Study the drawing (mm; zero at the part's minimum x, y, z) and answer. Round coordinates to 2 decimals unless told otherwise and drop trailing zeros. Write each loop counter-clockwise with the first axis right and the second up, starting at its lowest first coordinate (ties: lowest second). Pieces come first, ordered by that corner, then holes. Notation, with made-up numbers: (67.25, -1.75) - (104.25, -1.75) arc R26 cw to (104.25, 33.25) - close; hole circle Ø4 at (51.25, -38.75). An arc over 180 degrees is marked (long way). Return JSON: item names as keys, results as strings. Group by question number.
(1) Section B-B, the plane z = 48.5 is taken. Write down the section's boundary in (x, y), then the cut area to 3 significant figures.
(2) Find the intervals of material crossed by line 1 along Z through (x, y) = (15.25, 1.5); line 2 along X through (y, z) = (0.75, 15); line 3 along Y through (x, z) = (4.75, 224), in increasing order. Write a range as [from, to].
(3) Section D-D, the plane z = 235 is taken. Write down the section's boundary in (x, y), then the cut area to 3 significant figures.
(4) Section A-A, the plane x = 5 is taken. Write down the section's boundary in (y, z).
(5) Section C-C, the plane y = 5.5 is taken. Write down the section's boundary in (x, z).
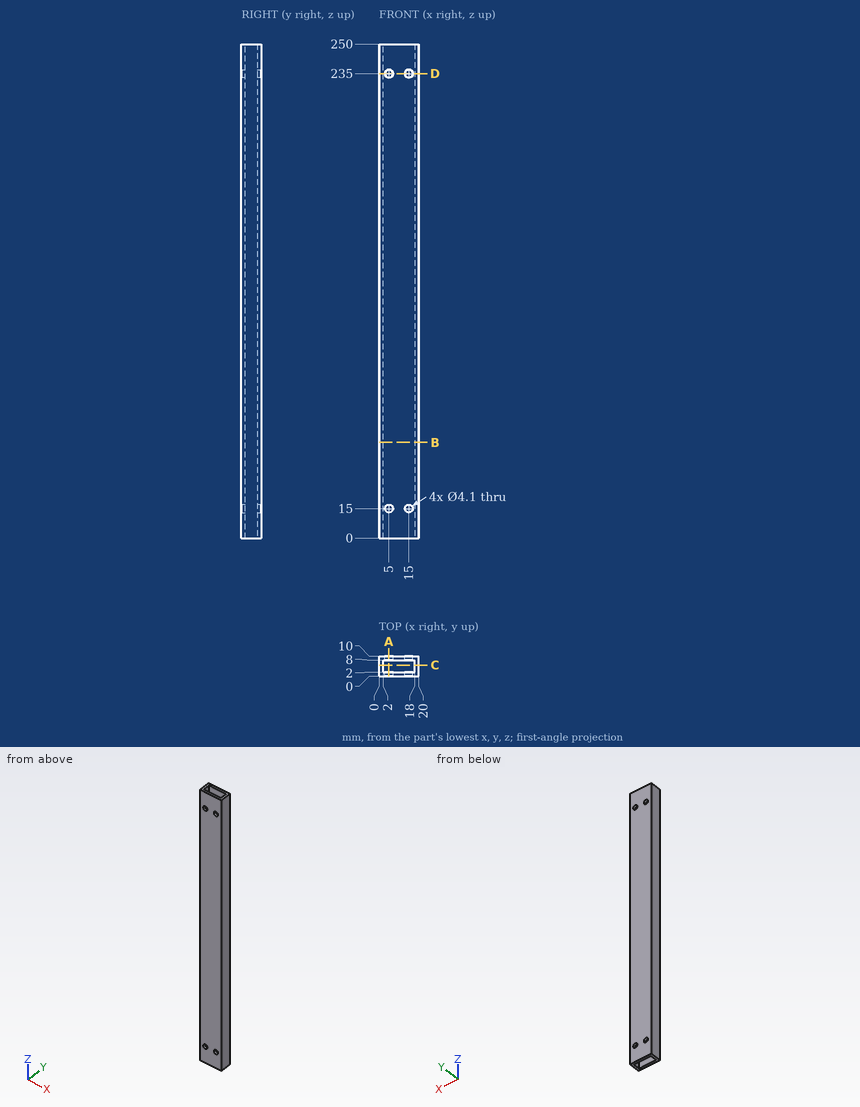
Working result:
{
 "1": {"outline": "(0, 0) - (20, 0) - (20, 10) - (0, 10) - close; hole (2, 2) - (18, 2) - (18, 8) - (2, 8) - close", "area": "104 mm^2"},
 "2": {"line 1": "z = [0, 12.97], [17.03, 232.97], [237.03, 250]", "line 2": "x = [0, 2.95], [7.05, 12.95], [17.05, 20]", "line 3": "y = [0, 2], [8, 10]"},
 "3": {"outline": "(0, 0) - (2.95, 0) - (2.95, 2) - (2, 2) - (2, 8) - (2.95, 8) - (2.95, 10) - (0, 10) - close; (7.05, 0) - (12.95, 0) - (12.95, 2) - (7.05, 2) - close; (7.05, 8) - (12.95, 8) - (12.95, 10) - (7.05, 10) - close; (17.05, 0) - (20, 0) - (20, 10) - (17.05, 10) - (17.05, 8) - (18, 8) - (18, 2) - (17.05, 2) - close", "area": "71.2 mm^2"},
 "4": {"outline": "(0, 0) - (2, 0) - (2, 12.95) - (0, 12.95) - close; (0, 17.05) - (2, 17.05) - (2, 232.95) - (0, 232.95) - close; (0, 237.05) - (2, 237.05) - (2, 250) - (0, 250) - close; (8, 0) - (10, 0) - (10, 12.95) - (8, 12.95) - close; (8, 17.05) - (10, 17.05) - (10, 232.95) - (8, 232.95) - close; (8, 237.05) - (10, 237.05) - (10, 250) - (8, 250) - close"},
 "5": {"outline": "(0, 0) - (2, 0) - (2, 250) - (0, 250) - close; (18, 0) - (20, 0) - (20, 250) - (18, 250) - close"}
}
